from build123d import *


with BuildPart() as part:
    # Esboço1 → Revolução1 (revolve)
    with BuildSketch(Plane.XY):
        Polygon((-27.999975, 5), (-27.999975, 16), (-28.699975, 16), (-28.699975, 10), (-30.399975, 10), (-30.399975, 16), (-31.099975, 16), (-31.099975, 10), (-32.799975, 10), (-32.799975, 16), (-33.499975, 16), (-33.499975, 10), (-35.199975, 10), (-35.199975, 16), (-35.899975, 16), (-35.899975, 10), (-37.599975, 10), (-37.599975, 16), (-38.299975, 16), (-38.299975, 10), (-39.999975, 10), (-39.999975, 16), (-40.699975, 16), (-40.699975, 10), (-42.399975, 10), (-42.399975, 16), (-43.099975, 16), (-43.099975, 10), (-44.799975, 10), (-44.799975, 16), (-45.499975, 16), (-45.499975, 10), (-47.199975, 10), (-47.199975, 16), (-47.899975, 16), (-47.899975, 10), (-49.599975, 10), (-49.599975, 16), (-50.299975, 16), (-50.299975, 10), (-51.999975, 10), (-51.999975, 16), (-52.699975, 16), (-52.699975, 10), (-54.399975, 10), (-54.399975, 12.9), (-55.099975, 12.9), (-55.099975, 10), (-56.799975, 10), (-56.799975, 12.9), (-59.799975, 12.9), (-59.799975, 10.9), (-65.799975, 10.9), (-65.799975, 12.9), (-69.099975, 12.9), (-69.099975, 5), align=None)
    revolve(axis=Axis((-27.999975, 5, 0), (-1, 0, 0)))


solid = part.part
Can you work these out from the model? Positions are in its coordinate system, mm. A direction names the side the tool comes from. Give positions to 0.01 mm unless a question says otherwise; leave off trailing zeros. Order: outer loops, then holes, each group sorted by start corner. A loop starts at its lowest first (then second) coordinate and runs counter-clockwise, first axis right, second up. Notation, with made-up numbers: (-32, -8.5) - (21, -8.5) arc R14 ccw to (21, 15.5) - close; hole circle Ø9 at (-9, 5). An arc over 180 degrees is marked (long way). Write each question's results on one line, items separated by ' | '.
1) Suppose I cut it at D-D, the plane x = -36.5. Write out the boundary of the cut face in (y, z).
Final values:
outline: circle Ø10 at (5, 0)
2) Suppose I cut it at A-A, the plane y = 14.25. Give the number of separate pieces and of enclosed holes in the cut face, then the cut area to 3 significant figures.
Final values:
separate pieces: 11 | enclosed holes: 0 | area: 91.7 mm^2
3) Please list where these lines run through material, in increasing order: line 1 along Y through (x, z) = (-35.5, -1.75); line 2 along Z through (x, y) = (-50, -2.5); line 3 along Z through (x, y) = (-62, 8.75). Write a range as [from, to].
Final values:
line 1: y = [-5.86, 15.86] | line 2: z = [-8.05, 8.05] | line 3: z = [-4.55, 4.55]
4) On a 3-axis mill with a long thin cutter (end or side, diameter ignored), from which of +Z, -Z, +X, -X, +Y, -Y can I reach the whole of each face in a straight line? I mean faces 1 (the face through (-52.35, 2.62, 10.74)), 2 (the face through (-45.5, 7, 5)). Say none if no direction works.
Final values:
face 1: +X, -X | face 2: none
5) I'm going to push flat-ended pins straight in: pin 1 Ø6 at (x, y) = (-63.5, -2.5) entering from +Z; pin 2 Ø3 at (x, z) = (-39, 8.5) entering from +Y; pin 3 Ø1.5 at (x, y) = (-63, 9) entering from -Z. Where does each tip first touch, or does it pass through?
Final values:
pin 1: stops at z = 5.6 | pin 2: stops at y = 13.34 | pin 3: stops at z = -4.92
6) If we mould it in two halves opening along X, with no side actions, what happens to faces 3 (the face through (-49.95, 2.62, 10.74)), 4 (the face through (-39, 0, 0))? For each: pulls with the +X half, pulls with the -X half, needs draft (parallel to the pull), parting line crosses it, or undercut.
Final values:
face 3: needs draft | face 4: undercut
7) Suppose I cut it at B-B, the plane x = -64.5. Write out the boundary of the cut face in (y, z), then the cut area to 3 significant figures.
Final values:
outline: circle Ø11.8 at (5, 0) | area: 109 mm^2
